The drawing under review shows one solid part. Ordinate dimensions are in mm from its lowest x, y, z. A direction names the side the tool comes from. Round coordinates to 2 decimals unless told otherwise and drop trailing zeros. Write each loop counter-clockwise with the first axis right and the second up, starting at its lowest first coordinate (ties: lowest second). Pieces come first, ordered by that corner, then holes. Notation, with made-up numbers: M 87.25,59 L 141.25,59 A29 ccw 141.25,80 Z; hole C 9,1.5 d4. An arc over 180 degrees is marked long. One line per item, written item: value. Start each with the question number.
1) Take a section at D-D, the plane x = 33. Write out the cut boundary in (y, z) (3 decimals).
2) Mouldability with a two-part tool opening along Z and no side actions: class the marked faces 1, 2 and 3 as +Z half, -Z half, draft (parallel to the pull), parting line (faces both ways), or undercut.
3) Take a section at C-C, the plane x = 3. Write out the cut boundary in (y, z).
4) For P1, Ø6, axis at x = 29, z = 71.5, coming from the +Y side; P2, Ø8, axis at x = 16, z = 93.5, coming from the -Y side; P3, Ø12, axis at y = 38.56, z = 60, coming from the -X side; P4, Ø4, axis at y = 21.56, z = 60, coming from the +X side, all flat-tipped, find the tip position at first contact; note any pin that passes through.
5) Tool access review of the marked faces 4, 5, 6 and 7: name each direction out of +Z, -Z, +X, -X, +Y, -Y from which nothing blocks a thin tool from reaching the whole face with its end or side.
6) Take a section at B-B, the plane y = 30.06. Write out the cut boundary in (x, z) (3 decimals), and give its area (4 significant figures).
7) Take a section at A-A, the plane z = 60. State how many separate pieces and enclosed holes the cut face has, and give its area (3 significant figures).
8) Wall thickness on probe 1 along Y at (x, z) = (35, 60) (3 decimals); probe 2 along Z at (x, y) = (29, 38); probe 3 along Y at (x, z) = (34.25, 60) (3 decimals): over which ranges is each line inside the solid? List them lowest first.
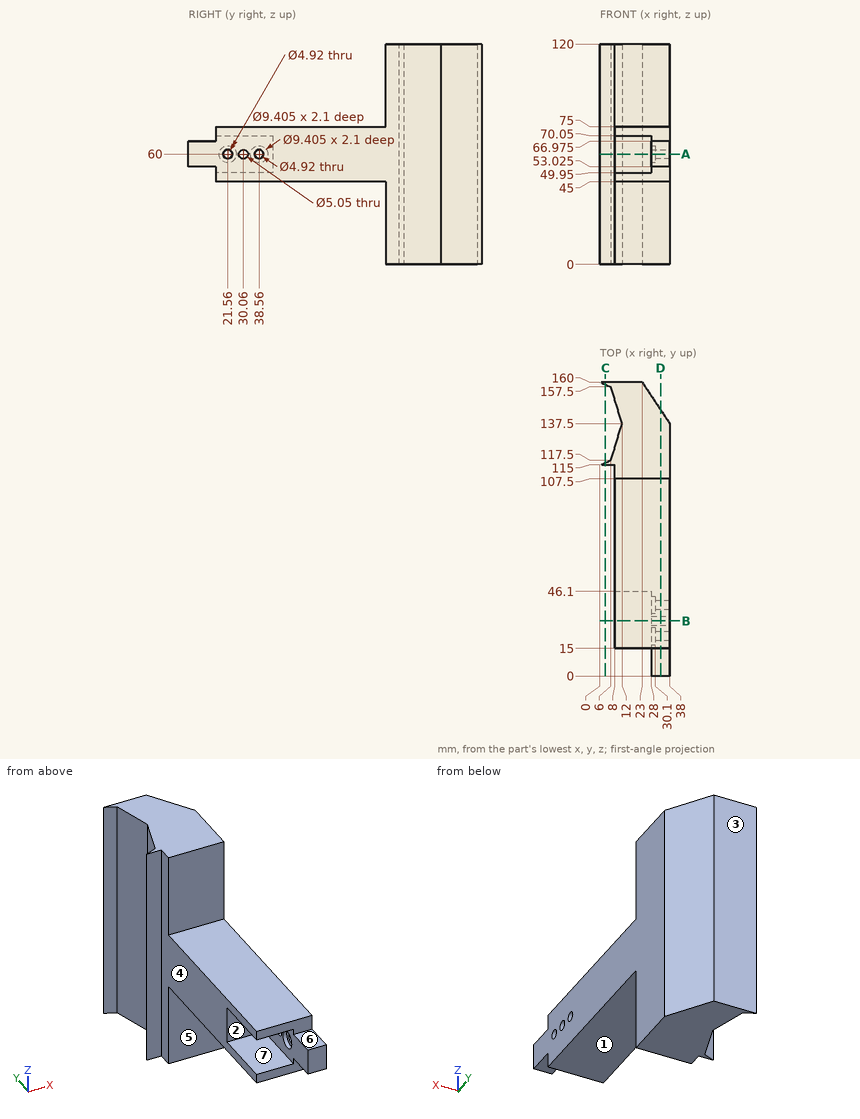
Checked values:
1. outline: M 0,53.025 L 15,53.025 L 15,45 L 107.5,45 L 107.5,0 L 145,0 L 145,120 L 107.5,120 L 107.5,75 L 15,75 L 15,66.975 L 0,66.975 Z; hole C 21.56,60 d4.92; hole C 30.06,60 d5.05; hole C 38.56,60 d4.92
2. face 1: -Z half
2. face 2: undercut
2. face 3: draft
3. outline: M 115,0 L 116.25,0 L 116.25,120 L 115,120 Z; M 158.75,0 L 160,0 L 160,120 L 158.75,120 Z
4. P1: stops at y = 155.5
4. P2: stops at y = 107.5
4. P3: stops at x = 28
4. P4: passes through
5. face 4: +Z, -Z, -X, -Y
5. face 5: -Z, +X, -X, -Y
5. face 6: +Z, +X, -X, -Y
5. face 7: -X, -Y
6. outline: M 8,45 L 38,45 L 38,57.475 L 28,57.475 L 28,49.95 L 8,49.95 Z; M 8,70.05 L 28,70.05 L 28,62.525 L 38,62.525 L 38,75 L 8,75 Z
6. area: 447.5 mm2
7. separate pieces: 4
7. enclosed holes: 0
7. area: 3,530 mm2
8. probe 1: y = 0 to 19.1, 24.02 to 27.535, 32.585 to 36.1, 41.02 to 142
8. probe 2: z = 45 to 55.33, 64.67 to 75
8. probe 3: y = 0 to 19.1, 24.02 to 27.535, 32.585 to 36.1, 41.02 to 143.125
